Verification items for the finished model (mm, model axes). Face numbers are marked on the shaded views. Give positions to 0.01 mm unless a question says otherwise; leave off trailing zeros. Loops run counter-clockwise (first coordinate to the right, second up) from the corner with the lowest first, then second, coordinate; pieces in that order, holes last. Notation, with made-up numbers: (62, 16) - (97, 16) arc R17 cw to (97, 45) - close; hole circle Ø11 at (22.25, 12.5). An arc over 180 degrees is marked (long way). One line per item, written item: value. Start each with the question number.
1. Sectioned sample at B-B (x = 57.5). Record the cut outline in (y, z), plus the area to 3 significant figures.
2. Gauge pin test, flat ends, axial feed: pin 1 (0.6 mm diameter, centred on x = 60.5, y = 1, fed in from -Z); pin 2 (5 mm diameter, centred on x = 42.5, z = -9, fed in from -Y). Record the tip position at first contact, or that the pin passes through.
3. Mould release check, pull along Y, two halves, no side actions. Record for the marked faces 1 and 2: pulls with the +Y half, pulls with the -Y half, needs draft (parallel to the pull), parting line crosses it, or undercut.
4. Scan lines: L1, parallel to Z at x = 55, y = 0.2; L2, parallel to X at y = 0.8, z = 35. Record each from-to range of solid material in increasing order. Write a range as [from, to].
5. Sectioned sample at A-A (y = 1.5). Record the cut outline in (x, z), plus the area to 3 significant figures.
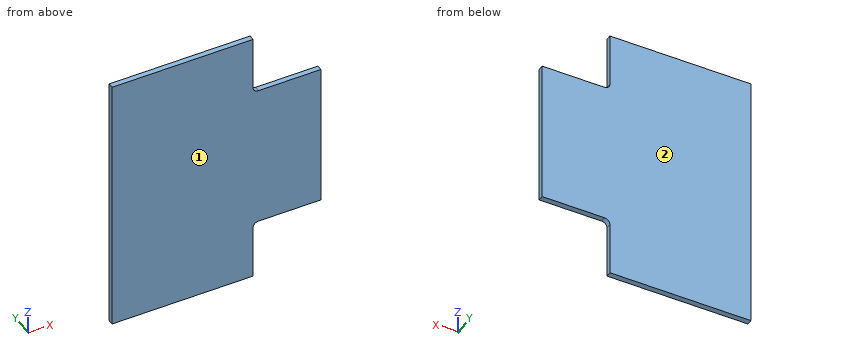
from build123d import *

# Parameters (mm, degrees)
SALIENTE_EXTRUIR1_DEPTH = 2


with BuildPart() as part:
    # Croquis1 → Saliente-Extruir1 (new body)
    with BuildSketch(Plane(origin=(0, 0, 0), x_dir=(1, 0, 0), z_dir=(0, 1, 0))):
        with BuildLine():
            Line((0, -49), (0, 49))
            Line((0, 49), (52, 49))
            Line((52, 49), (52, 29))
            ThreePointArc((52, 29), (52.585786438, 27.585786438), (54, 27))
            Line((54, 27), (77, 27))
            Line((77, 27), (77, -27))
            Line((77, -27), (54, -27))
            ThreePointArc((54, -27), (52.585786438, -27.585786438), (52, -29))
            Line((52, -29), (52, -49))
            Line((52, -49), (0, -49))
        make_face()
    extrude(amount=SALIENTE_EXTRUIR1_DEPTH)


solid = part.part
Results are:
1. outline: (0, -27) - (2, -27) - (2, 27) - (0, 27) - close
1. area: 108 mm^2
2. pin 1: stops at z = -27
2. pin 2: stops at y = 0
3. face 1: pulls with the -Y half
3. face 2: pulls with the +Y half
4. L1: z = [-27, 27]
4. L2: x = [0, 52]
5. outline: (0, -49) - (52, -49) - (52, -29) arc R2 cw to (54, -27) - (77, -27) - (77, 27) - (54, 27) arc R2 cw to (52, 29) - (52, 49) - (0, 49) - close
5. area: 6,450 mm^2
